Autodesk Inventor part; units mm, degrees
ref_plane "YZ Plane" through (0, 0, 0) normal (1, 0, 0) x (0, 1, 0)
ref_plane "XZ Plane" through (0, 0, 0) normal (0, 1, 0) x (-1, 0, 0)
ref_plane "XY Plane" through (0, 0, 0) normal (0, 0, 1) x (1, 0, 0)
ref_plane "Work Plane1" through (-12.7, 499.15, -25.4) normal (0, 1, 0) x (-1, 0, 0)
sketch "Sketch1" plane through (-12.7, 499.15, -25.4) normal (0, 1, 0) x (-1, 0, 0)
  line L0 (-19.05, 819.05) -> (-19.05, -19.05)
  line L1 (-12.7, 35.4) -> (-2.7, 35.4)
  line L2 (-12.7, 764.6) -> (-2.7, 764.6)
  line L3 (-19.05, 25.4) -> (105.4044, 25.4)
  line L4 (105.4044, 25.4) -> (105.4044, 774.6084)
  line L5 (105.4044, 774.6084) -> (-19.05, 774.6084)
  line L6 (-19.05, 774.6084) -> (-19.05, 25.4)
  point P0 (-12.7, 25.4)
  point P1 (-19.05, 774.6084)
  dimension "d0" = 749.2084
  dimension "d1" = 124.4544
extrude "Extrusion1" add sketch "Sketch1" along normal blind 661.25
ref_plane "Work Plane2" through (6.35, 499.15, 793.65) normal (0.766, -0.6428, 0) x (0, 0, -1)
sketch "Sketch2" plane through (6.35, 499.15, 793.65) normal (0.766, -0.6428, 0) x (0, 0, -1)
  line L0 (44.4416, 0) -> (44.4416, 506.5469)
  line L1 (44.4416, 167.8683) -> (793.65, 167.8683)
  line L2 (793.65, 167.8683) -> (793.65, -166.4116)
  line L3 (793.65, -166.4116) -> (44.4416, -166.4116)
  line L4 (44.4416, -166.4116) -> (44.4416, 167.8683)
  point P0 (793.65, -386.4528)
extrude "Extrusion2" cut sketch "Sketch2" against normal blind 96.5
shell "Shell1" thickness 5 removed faces 1 at (-35.1348, 599.8377, 499.4722)
properties part number "DUSTPAN" material "Polystyrene"
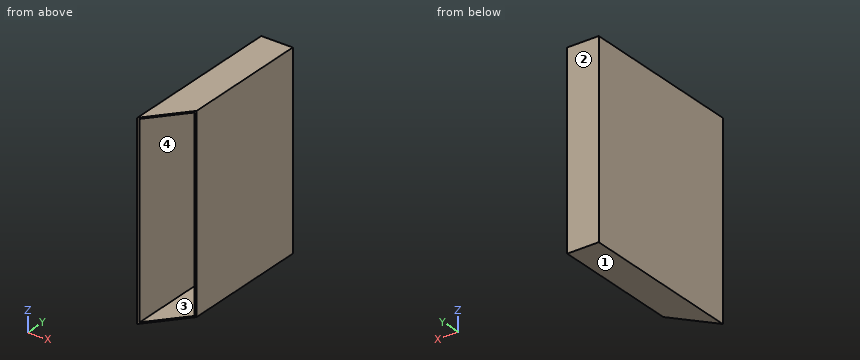
Could you check a few things on this model? Use its own coordinates, in mm. Face numbers are marked on the shaded views. Coordinates: 2 decimals unless noted, no trailing zeros. Write each loop counter-clockwise with the first axis right and the second up, starting at its lowest first coordinate (ties: lowest second). Pieces come first, ordered by that corner, then holes. Notation, with made-up numbers: (51.25, -19) - (89.25, -19) arc R20 ccw to (89.25, -13) - close; hole circle Ø11 at (22.25, -39.5). An arc over 180 degrees is marked (long way). Put each result on its own line as item: value. Start each with the question number.
Q1. I'm going to push a flat-ended pin straight in: P1, Ø1.5, axis at x = -62, z = 494, coming from the -Y side. Where does the tip first touch, or does it pass through?
Q2. Please list where these lines run through material, in increasing order: L1, parallel to Z at x = -38.5, y = 889.5; L2, parallel to X at y = 1098, z = 439.5; L3, parallel to Y at x = -94.5, z = 348.5.
Q3. I want a section at B-B on z = 329. Write out the boundary of the cut face in (x, y), plus the area to 3 significant figures.
Q4. I want a section at A-A on y = 1026.5. Write out the boundary of the cut face in (x, z).
Q5. Thinking about a two-plate mould opening in Z: for the marked faces 1, 2, 3 and 4, which applies, pulls with the +Z half, pulls with the -Z half, needs draft (parallel to the pull), parting line crosses it, or undercut?
Q6. I want a section at C-C on x = -73.5. Write out the boundary of the cut face in (y, z), plus the area to 3 significant figures.
Checks:
1. P1: y = 1155.4
2. L1: 0 to 5, 744.21 to 749.21
2. L2: -118.1 to -113.1, 1.35 to 6.35
2. L3: 1155.4 to 1160.4
3. outline: (-118.1, 500.96) - (-113.1, 506.92) - (-113.1, 1155.4) - (1.35, 1155.4) - (1.35, 643.32) - (6.35, 649.28) - (6.35, 1160.4) - (-118.1, 1160.4) - close
3. area: 6,430 mm²
4. outline: (-118.1, 0) - (6.35, 0) - (6.35, 749.21) - (-118.1, 749.21) - close; hole (-113.1, 5) - (1.35, 5) - (1.35, 744.21) - (-113.1, 744.21) - close
5. face 1: pulls with the -Z half
5. face 2: needs draft
5. face 3: undercut
5. face 4: undercut
6. outline: (554.12, 0) - (1160.4, 0) - (1160.4, 749.21) - (554.12, 749.21) - (554.12, 744.21) - (1155.4, 744.21) - (1155.4, 5) - (554.12, 5) - close
6. area: 9,760 mm²
